Autodesk Inventor part; units mm, degrees
ref_plane "Work Plane1" through (0, -6, 184.2137) normal (-1, 0, 0) x (0, 0, 1)
ref_plane "YZ Plane" through (0, 0, 0) normal (1, 0, 0) x (0, 1, 0)
ref_plane "XZ Plane" through (0, 0, 0) normal (0, 1, 0) x (-1, 0, 0)
sketch "Tube Base Sketch" plane through (0, 0, 0) normal (0, 0, 1) x (1, 0, 0)
  line L0 (-5, -5) -> (5, -5)
  line L1 (5, -5) -> (5, 5)
  line L2 (5, 5) -> (-5, 5)
  line L3 (-5, 5) -> (-5, -5)
  line L4 (-5, -5) -> (5, 5) construction
  line L5 (5, -5) -> (-5, 5) construction
  line L6 (-6, 6) -> (6, 6)
  line L7 (6, 6) -> (6, -6)
  line L8 (6, -6) -> (-6, -6)
  line L9 (-6, -6) -> (-6, 6)
  point P0 (0, 0)
  dimension "TubeWidth" = 10
  dimension "TubeHeight" = 10
  dimension "WallThickness" = 1
extrude "Tube" add sketch "Tube Base Sketch" along normal blind 184.2137
sketch "Cap Sketch" plane through (0, 0, 0) normal (0, 0, -1) x (-1, 0, 0)
  line L0 (-6, -6) -> (6, -6)
  line L1 (6, -6) -> (6, 8)
  line L2 (6, 8) -> (-6, 8)
  line L3 (-6, 8) -> (-6, -6)
  point P0 (0, 0)
  dimension "CapHeight" = 14
extrude "Extrusion6" add sketch "Cap Sketch" along normal blind 20
ref_plane "Work Plane1" through (0, -6, 184.2137) normal (-1, 0, 0) x (0, 0, 1)
sketch "Edge Cut and Slit Sketch" plane through (0, -6, 184.2137) normal (-1, 0, 0) x (0, 0, 1)
  line L0 (-184.2137, 12) -> (0, 12)
  line L1 (-184.2137, 11) -> (-184.2137, 1) construction
  line L2 (-184.2137, 12) -> (-184.2137, 10) construction
  line L3 (-184.2137, 10) -> (-169.2137, 12)
  line L4 (-204.2137, 0) -> (-204.2137, 14)
  line L5 (-184.2137, 12) -> (-204.2137, 12)
  line L6 (-184.2137, 10) -> (-204.2137, 10)
  point P0 (-184.2137, 6)
  dimension "EdgeCutDepth" = 2
  dimension "EdgeCutLength" = 15
extrude "Edge Cut and Slit" cut sketch "Edge Cut and Slit Sketch" along normal mid plane 8
equation "\"TubeWidth\" = MaxWidth"
equation "\"TubeHeight\" = TubeWidth"
equation "\"TubeLength\" = DesiredLength + PlugLength"
equation "\"EdgeCutDepth\" = 2 * WallThickness"
equation "\"d26\" = TubeWidth - 2 * WallThickness"
equation "\"MaxWidth\" = 10"
equation "\"DesiredLength\" = 164.21369"
equation "\"PlugLength\" = 20"
properties part number "Whistle1"
Read the model definition and answer for the solid it produces. Units are mm, in the model's axes. A direction names the side the tool comes from. Give positions to 0.01 mm unless a question says otherwise; leave off trailing zeros. Write each loop counter-clockwise with the first axis right and the second up, starting at its lowest first coordinate (ties: lowest second). Pieces come first, ordered by that corner, then holes. Notation, with made-up numbers: (-30.75, 60) -> (1.25, 60) arc R18 cw to (1.25, 74) -> close; hole circle Ø2 at (-30, 3.25). An arc over 180 degrees is marked (long way). Answer in a Markdown table with one row per item.
1) Section C-C on y = -2.75 is taken. Give the vertices of the cut face in (x, z).
Results list:
| item | result |
|---|---|
| outline | (-6, -20) -> (6, -20) -> (6, 184.21) -> (5, 184.21) -> (5, 0) -> (-5, 0) -> (-5, 184.21) -> (-6, 184.21) -> close |
2) Section A-A on x = -0.25 is taken. Give the vertices of the cut face in (y, z).
Results list:
| item | result |
|---|---|
| outline | (-6, -20) -> (4, -20) -> (4, 0) -> (-5, 0) -> (-5, 184.21) -> (-6, 184.21) -> close; (5, 7.5) -> (6, 15) -> (6, 184.21) -> (5, 184.21) -> close; (6, -20) -> (8, -20) -> (8, 0) -> (6, 0) -> close |
3) Determine the mould class of faces 4 (the flat face through (0, -5, 91)), 5 (the flat face through (0, 6, 91)), 6 (the flat face through (-6, 1, 81)) for opening direction X: released by +X, released by -X, zero draft, split by the parting line, or undercut.
Results list:
| item | result |
|---|---|
| face 4 | undercut |
| face 5 | zero draft |
| face 6 | released by -X |
4) Each of these flat-tipped pins is pushed along its axis until it touches: pin 1 Ø3 at (x, y) = (2, 1) entering from +Z; pin 2 Ø2 at (x, z) = (0, 119.5) entering from +Y. Where does it stop, or does it pass through?
Results list:
| item | result |
|---|---|
| pin 1 | z = 0 |
| pin 2 | y = 6 |
5) Straight lines are drawn through the part: line 1 (Y direction, x = -2.5, z = 60.5); line 2 (Z direction, x = -4, y = -1.5). For each, find the intervals that lie inside material, in ascending order. Write a range as [from, to].
Results list:
| item | result |
|---|---|
| line 1 | [-6, -5], [5, 6] |
| line 2 | [-20, 0] |
6) Section B-B on z = 107 is taken. Give the vertices of the cut face in (x, y), plus the area to 3 significant figures.
Results list:
| item | result |
|---|---|
| outline | (-6, -6) -> (6, -6) -> (6, 6) -> (-6, 6) -> close; hole (-5, -5) -> (5, -5) -> (5, 5) -> (-5, 5) -> close |
| area | 44.0 mm^2 |
7) A tool of negligible diameter and unlimited length cuts with its end or side. For faces 1 (the flat face through (0, 4, -10)), 2 (the flat face through (5, 0, 91)), 3 (the flat face through (0, 6, -10)), from which of +Z, -Z, +X, -X, +Y, -Y can it reach the whole face along a straight path? Write none if from no direction.
Results list:
| item | result |
|---|---|
| face 1 | +Z, -Z |
| face 2 | +Z |
| face 3 | -Z |
